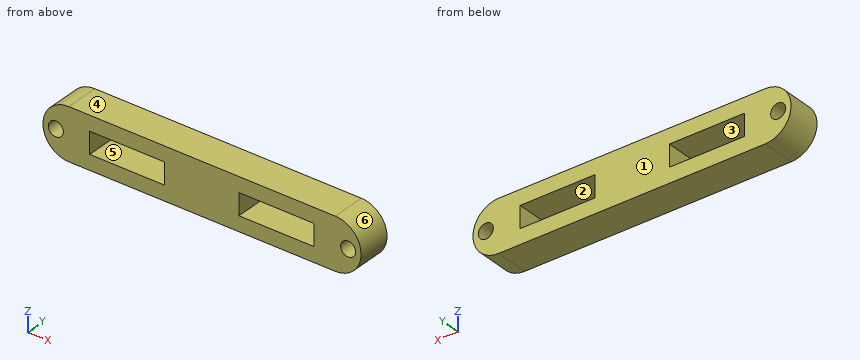
```python
from build123d import *

# Parameters (mm, degrees)
SKETCH1_W                = 22.609360872
SKETCH1_H                = 4.3815
SKETCH1_W_2              = 6.35
SKETCH1_H_2              = 1.8415
BOSS_EXTRUDE1_DEPTH      = 6.35
BOSS_EXTRUDE2_REACH      = 15.15
BOSS_EXTRUDE3_START      = 2.19075
BOSS_EXTRUDE3_DEPTH      = 2.19075
SKETCH7_R                = 1.5875
BOSS_EXTRUDE4_DEPTH      = 1.27
MIRROR2_COPY_1_SKETCH_R  = 1.5875
MIRROR2_COPY_1_DEPTH     = 1.27
BOSS_EXTRUDE5_DEPTH      = 6.35
BOSS_EXTRUDE5_DEPTH_BACK = 1.27
SKETCH8_R                = 0.635
SKETCH9_W                = 22.609360872
SKETCH9_H                = 6.35
BOSS_EXTRUDE6_DEPTH      = 4.3815
SKETCH10_W               = 6.35
SKETCH10_H               = 1.8415
CUT_EXTRUDE1_DEPTH       = 12.7
CUT_EXTRUDE2_DEPTH       = 23.114
CUT_EXTRUDE2_DEPTH_BACK  = 4.7625
SKETCH12_W               = 31.633822951
SKETCH12_H               = 14.456952732


with BuildPart() as part:
    # Sketch1 → Boss-Extrude1 (new body)
    with BuildSketch(Plane(origin=(0, 0, 0), x_dir=(1, 0, 0), z_dir=(0, 1, 0))):
        Rectangle(SKETCH1_W, SKETCH1_H)
        with Locations((-6.35, 0)):
            Rectangle(SKETCH1_W_2, SKETCH1_H_2, mode=Mode.SUBTRACT)
        with Locations((6.308703221, 0)):
            Rectangle(SKETCH1_W_2, SKETCH1_H_2, mode=Mode.SUBTRACT)
    extrude(amount=BOSS_EXTRUDE1_DEPTH)

    # Boss-Extrude2: up to this face of the body (flat: up to its plane)
    boss_extrude2_end = Plane(part.part.faces().sort_by_distance((0, 3.175, -2.19075))[0])
    # Sketch2 → Boss-Extrude2 (add, up to the picked face)
    with BuildSketch(Plane.XY, mode=Mode.PRIVATE) as boss_extrude2_sk1:
        with BuildLine():
            Line((3.175, 0), (-3.175, 0))
            ThreePointArc((-3.175, 0), (0, -3.175), (3.175, 0))
        make_face()
    boss_extrude2_tool1 = split(extrude(boss_extrude2_sk1.sketch, amount=-BOSS_EXTRUDE2_REACH, mode=Mode.PRIVATE), bisect_by=boss_extrude2_end, keep=Keep.BOTH, mode=Mode.PRIVATE)
    add(boss_extrude2_tool1.solids().sort_by(Axis((0, -1.347512, 0), (0, 0, -1)))[0])

    # Sketch2<3> → Boss-Extrude3 (add)
    with BuildSketch(Plane.XY.offset(BOSS_EXTRUDE3_START)):
        with BuildLine():
            Line((3.175, 0), (-3.175, 0))
            ThreePointArc((-3.175, 0), (0, -3.175), (3.175, 0))
        make_face()
    extrude(amount=-BOSS_EXTRUDE3_DEPTH)

    # Sketch7 → Boss-Extrude4 (add)
    with BuildSketch(Plane.XY.offset(2.19075)):
        with BuildLine():
            Line((-9.525, 0), (-11.304680436, 0))
            Line((-11.304680436, 0), (-11.304680436, -12.7))
            ThreePointArc((-11.304680436, -12.7), (-8.266575896, -13.958424104), (-9.525, -10.920319564))
            Line((-9.525, -10.920319564), (-9.525, 0))
        make_face()
        with Locations((-9.525, -12.7)):
            Circle(SKETCH7_R, mode=Mode.SUBTRACT)
    boss_extrude4 = extrude(amount=-BOSS_EXTRUDE4_DEPTH)

    # Mirror1: Boss-Extrude4 across plane
    add(boss_extrude4.mirror(Plane(origin=(0, 0, 0), x_dir=(0, 0, 1), z_dir=(1, 0, 0))))

    # Mirror2: Boss-Extrude4 across plane
    add(boss_extrude4.mirror(Plane.XY))

    # Mirror2 copy 1 sketch → Mirror2 copy 1 (add)
    with BuildSketch(Plane(origin=(0, 0, -2.19075), x_dir=(-1, 0, 0), z_dir=(0, 0, -1))):
        with BuildLine():
            Line((-9.525, 0), (-11.304680436, 0))
            Line((-11.304680436, 0), (-11.304680436, -12.7))
            ThreePointArc((-11.304680436, -12.7), (-8.266575896, -13.958424104), (-9.525, -10.920319564))
            Line((-9.525, -10.920319564), (-9.525, 0))
        make_face()
        with Locations((-9.525, -12.7)):
            Circle(MIRROR2_COPY_1_SKETCH_R, mode=Mode.SUBTRACT)
    extrude(amount=-MIRROR2_COPY_1_DEPTH)

    # Sketch8 → Boss-Extrude5 (add, two sides: drawn at the far end of the back side and taken through both)
    # profile 1 of 2: a face of its own
    with BuildSketch(Plane(origin=(0, 6.35, 0), x_dir=(1, 0, 0), z_dir=(0, 1, 0)).offset(-BOSS_EXTRUDE5_DEPTH_BACK)):
        with BuildLine():
            Line((-11.304680436, 2.19075), (-11.304680436, -2.19075))
            ThreePointArc((-11.304680436, -2.19075), (-13.495430436, 0), (-11.304680436, 2.19075))
        make_face()
        with Locations(Location((-12.400055436, 0, 0), (0, 0, 270))):
            Circle(SKETCH8_R, mode=Mode.SUBTRACT)
    # profile 2 of 2: a face of its own
    with BuildSketch(Plane(origin=(0, 6.35, 0), x_dir=(1, 0, 0), z_dir=(0, 1, 0)).offset(-BOSS_EXTRUDE5_DEPTH_BACK)):
        with BuildLine():
            Line((11.304680436, 2.19075), (11.304680436, -2.19075))
            ThreePointArc((11.304680436, -2.19075), (13.495430436, 0), (11.304680436, 2.19075))
        make_face()
        with Locations(Location((12.400055436, 0, 0), (0, 0, 90))):
            Circle(SKETCH8_R, mode=Mode.SUBTRACT)
    extrude(amount=BOSS_EXTRUDE5_DEPTH + BOSS_EXTRUDE5_DEPTH_BACK)

    # Sketch9 → Boss-Extrude6 (add)
    with BuildSketch(Plane(origin=(0, 0, -2.19075), x_dir=(-1, 0, 0), z_dir=(0, 0, -1))):
        with Locations((0, 9.525)):
            Rectangle(SKETCH9_W, SKETCH9_H)
    extrude(amount=-BOSS_EXTRUDE6_DEPTH)

    # Sketch10 → Cut-Extrude1 (cut)
    with BuildSketch(Plane(origin=(0, 12.7, 0), x_dir=(1, 0, 0), z_dir=(0, 1, 0))):
        with Locations((6.308703221, 0)):
            Rectangle(SKETCH10_W, SKETCH10_H)
        with Locations((-6.35, 0)):
            Rectangle(SKETCH10_W, SKETCH10_H)
    extrude(amount=-CUT_EXTRUDE1_DEPTH, mode=Mode.SUBTRACT)

    # Sketch12 → Cut-Extrude2 (cut, two sides: drawn at the far end of the back side and taken through both)
    with BuildSketch(Plane(origin=(0, 5.08, 0), x_dir=(-1, 0, 0), z_dir=(0, -1, 0)).offset(-CUT_EXTRUDE2_DEPTH_BACK)):
        with Locations((-0.08433307, 1.389523064)):
            Rectangle(SKETCH12_W, SKETCH12_H)
    extrude(amount=CUT_EXTRUDE2_DEPTH + CUT_EXTRUDE2_DEPTH_BACK, mode=Mode.SUBTRACT)


solid = part.part
```
Check sheet for the modelled part. Datum: model origin and axes. Units: mm. Face numbers are marked on the shaded views. A direction names the side the tool comes from. Coordinates: 2 decimals unless noted, no trailing zeros. Order: outer loops, then holes, each group sorted by start corner. A loop starts at its lowest first (then second) coordinate and runs counter-clockwise, first axis right, second up. Notation, with made-up numbers: (52, 7) -> (95, 7) arc R14 ccw to (95, 32) -> close; hole circle Ø7 at (-3, 19). An arc over 180 degrees is marked (long way). Write each question's results on one line, items separated by ' | '. Start each with the question number.
1) Section check B-B (x = -8.25). Enter the section's corners in (y, z).
2) Set-up check for the marked faces 1 and 2: record each of +Z, -Z, +X, -X, +Y, -Y from which the full face is reachable in a straight line by a thin tool's end or side.
3) Section check D-D (z = 1.9). Enter the section's corners in (x, y).
4) Section check A-A (z = 0). Enter the section's corners in (x, y) (1 decimal).
5) Draft check along X on the marked faces 3, 4, 5 and 6. Enter one of: pulls with the +X half, pulls with the -X half, needs draft (parallel to the pull), parting line crosses it, or undercut.
6) Section check C-C (y = 12.35). Enter the section's corners in (x, z) (1 decimal), and give its area (3 significant figures).
7) Depth check by flat-ended pin: pin 1 (1 mm diameter, centred on y = 12.5, z = 1, fed in from +X); pin 2 (1.5 mm diameter, centred on x = -4, z = 0.5, fed in from +Y); pin 3 (0.6 mm diameter, centred on y = 11, z = 0.5, fed in from +X). Enter the tip coordinate at first touch or a pass-through.
8) Material ranges on line 1 along X through (y, z) = (12.1, 0) (3 decimals); line 2 along Z through (x, y) = (3.5, 12.2); line 3 along X through (y, z) = (10.35, -0.5) (1 decimal), recorded low to high.
Checked values:
1) outline: (9.84, -2.19) -> (12.7, -2.19) -> (12.7, -0.92) -> (9.84, -0.92) -> close; (9.84, 0.92) -> (12.7, 0.92) -> (12.7, 2.19) -> (9.84, 2.19) -> close
2) face 1: +Z, -Z, +X, -X, +Y | face 2: +Y, -Y
3) outline: (-12.4, 9.84) -> (12.4, 9.84) -> (12.4, 12.7) -> (-12.4, 12.7) -> close
4) outline: (-13.5, 9.8) -> (-13, 9.8) -> (-13, 12.7) -> (-13.5, 12.7) -> close; (-11.8, 9.8) -> (-9.5, 9.8) -> (-9.5, 12.7) -> (-11.8, 12.7) -> close; (-3.2, 9.8) -> (3.1, 9.8) -> (3.1, 12.7) -> (-3.2, 12.7) -> close; (9.5, 9.8) -> (11.8, 9.8) -> (11.8, 12.7) -> (9.5, 12.7) -> close; (13, 9.8) -> (13.5, 9.8) -> (13.5, 12.7) -> (13, 12.7) -> close
5) face 3: undercut | face 4: needs draft | face 5: undercut | face 6: pulls with the +X half
6) outline: (-11.3, -2.2) -> (11.3, -2.2) arc R2.2 ccw to (11.3, 2.2) -> (-11.3, 2.2) arc R2.2 ccw to start; hole circle Ø1.3 at (-12.4, 0); hole (-9.5, -0.9) -> (-3.2, -0.9) -> (-3.2, 0.9) -> (-9.5, 0.9) -> close; hole (3.1, -0.9) -> (9.5, -0.9) -> (9.5, 0.9) -> (3.1, 0.9) -> close; hole circle Ø1.3 at (12.4, 0) | area: 88.2 mm²
7) pin 1: x = 13.44 | pin 2: y = 12.7 | pin 3: x = 13.49
8) line 1: -13.495 to -13.035, -11.765 to -9.525, -3.175 to 3.134, 9.484 to 11.765, 13.035 to 13.495 | line 2: -2.19 to -0.92, 0.92 to 2.19 | line 3: -13.4 to -12.8, -12 to -9.5, -3.2 to 3.1, 9.5 to 12, 12.8 to 13.4
